Model file for the job. Use its own axes, mm. Coordinates: 2 decimals unless noted, no trailing zeros. Loops run counter-clockwise (first coordinate to the right, second up) from the corner with the lowest first, then second, coordinate; pieces in that order, holes last. Notation, with made-up numbers: M 1.25,77.25 L 41.25,77.25 A22 cw 41.25,110.25 Z; hole C 71.25,-10.5 d10. An arc over 180 degrees is marked long. Write item = value, one per line. Start each with the question number.
from build123d import *

# Parameters (mm, degrees)
SALIENTE_EXTRUIR1_DEPTH = 3500
CROQUIS2_R              = 4.85898955
SALIENTE_EXTRUIR2_DEPTH = 24
CROQUIS3_W              = 61.744916595
CROQUIS3_H              = 103.748261218
CORTAR_EXTRUIR1_DEPTH   = 750
CROQUIS4_W              = 41.753180027
CROQUIS4_H              = 90.106519095
CORTAR_EXTRUIR2_DEPTH   = 750


with BuildPart() as part:
    # Croquis1 → Saliente-Extruir1 (new body)
    with BuildSketch(Plane.XY):
        Polygon((0, 0), (0, 80), (30, 80), (30, 77), (3, 77), (3, 3), (30, 3), (30, 0), align=None)
    extrude(amount=SALIENTE_EXTRUIR1_DEPTH)

    # Croquis2 → Saliente-Extruir2 (add)
    with BuildSketch(Plane(origin=(0, 0, 0), x_dir=(0, 0, -1), z_dir=(1, 0, 0))):
        with Locations((-1725, 20.15133135)):
            Circle(CROQUIS2_R)
        with Locations((-1725, 60.453994049)):
            Circle(CROQUIS2_R)
        with Locations((-1775, 20.15133135)):
            Circle(CROQUIS2_R)
        with Locations((-1775, 60.453994049)):
            Circle(CROQUIS2_R)
    extrude(amount=-SALIENTE_EXTRUIR2_DEPTH)

    # Croquis3 → Cortar-Extruir1 (cut)
    with BuildSketch(Plane.XY):
        with Locations((6.570284293, 36.219698984)):
            Rectangle(CROQUIS3_W, CROQUIS3_H)
    extrude(amount=CORTAR_EXTRUIR1_DEPTH, mode=Mode.SUBTRACT)

    # Croquis4 → Cortar-Extruir2 (cut)
    with BuildSketch(Plane.XY.offset(3500)):
        with Locations((13.937202, 38.995627971)):
            Rectangle(CROQUIS4_W, CROQUIS4_H)
    extrude(amount=-CORTAR_EXTRUIR2_DEPTH, mode=Mode.SUBTRACT)


solid = part.part
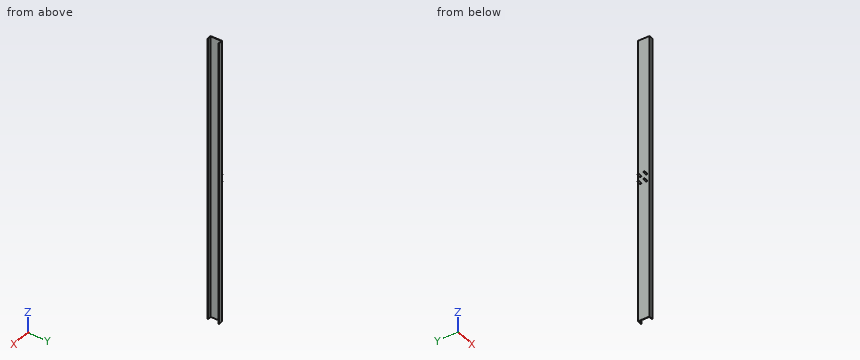
Item 1: Probe L1, parallel to Y at x = 13, z = 2253; L2, parallel to X at y = 55.5, z = 1848; L3, parallel to Z at x = -5, y = 64. List the from-to ranges inside material, lowest first.
Item 2: Cut at A-A (z = 2539). Give the cut face in (x, y), plus the area to 3 significant figures.
Item 3: Pin check, flat tips, straight feed: pin 1 Ø1 at (x, y) = (-2.5, 61.5) entering from +Z; pin 2 Ø3 at (y, z) = (38.5, 1236.5) entering from +X; pin 3 Ø4 at (y, z) = (65, 1220.5) entering from -X; pin 4 Ø10 at (x, z) = (9, 2300) entering from -Y. Stop position of each tip, or through.
Reported:
q1.L1 = 0 to 3, 77 to 80
q1.L2 = 0 to 3
q1.L3 = 1721.68 to 1728.32, 1771.68 to 1778.32
q2.outline = M 0,0 L 30,0 L 30,3 L 3,3 L 3,77 L 30,77 L 30,80 L 0,80 Z
q2.area = 402 mm^2
q3.pin_1 = 1779.83
q3.pin_2 = 3
q3.pin_3 = 0
q3.pin_4 = 0
